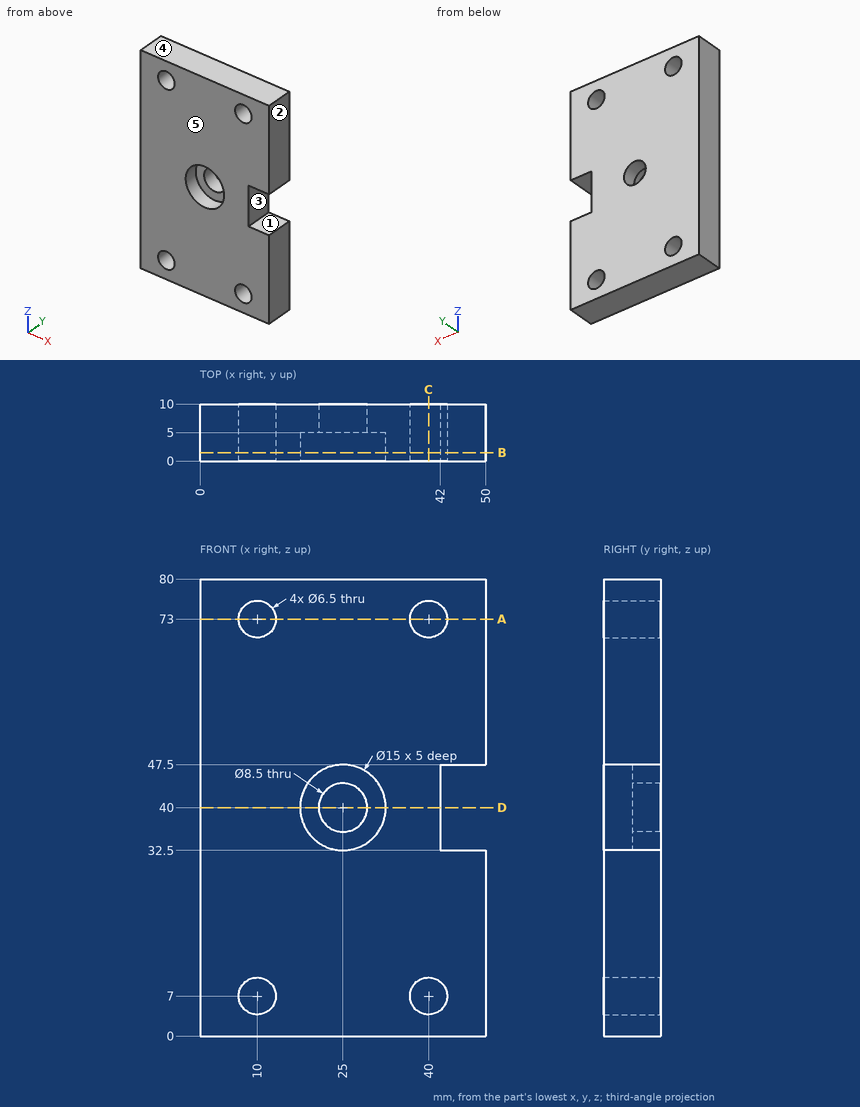
Geometry: see drawing. Coordinates: mm, zero at the bounding-box minimum. A direction names the side the tool comes from. Give positions to 0.01 mm unless a question says otherwise; leave off trailing zeros. Order: outer loops, then holes, each group sorted by start corner. A loop starts at its lowest first (then second) coordinate and runs counter-clockwise, first axis right, second up. Notation, with made-up numbers: (67, -37.75) - (71, -37.75) arc R20 ccw to (71, 0.25) - close; hole circle Ø9 at (-14, 79.25). An arc over 180 degrees is marked (long way). Use CSV: the item, a comma, the result in double quotes.
1. Section query D-D (z = 40). Output: boundary loops of the cut face in (x, y), plus the area to 4 significant figures.
Answers below:
outline,"(0, 0) - (17.5, 0) - (17.5, 5) - (20.75, 5) - (20.75, 10) - (0, 10) - close; (29.25, 5) - (32.5, 5) - (32.5, 0) - (42, 0) - (42, 10) - (29.25, 10) - close"
area,"302.5 mm2"
2. Section query B-B (y = 1.5). Output: boundary loops of the cut face in (x, z), plus the area to 3 significant figures.
Answers below:
outline,"(0, 0) - (50, 0) - (50, 32.5) - (42, 32.5) - (42, 47.5) - (50, 47.5) - (50, 80) - (0, 80) - close; hole circle Ø6.5 at (10, 7); hole circle Ø6.5 at (10, 73); hole circle Ø15 at (25, 40); hole circle Ø6.5 at (40, 7); hole circle Ø6.5 at (40, 73)"
area,"3,570 mm2"
3. Section query A-A (z = 73). Output: boundary loops of the cut face in (x, y), plus the area to 3 significant figures.
Answers below:
outline,"(0, 0) - (6.75, 0) - (6.75, 10) - (0, 10) - close; (13.25, 0) - (36.75, 0) - (36.75, 10) - (13.25, 10) - close; (43.25, 0) - (50, 0) - (50, 10) - (43.25, 10) - close"
area,"370 mm2"
4. Contact query for a flat-ended pin moving along its axis: pin 1 (13.5 mm diameter, centred on x = 25, z = 40, fed in from -Y). Output: stop coordinate, or through.
Answers below:
pin 1,"y = 5"
5. Mould query, pull axis Z, two halves, no side actions, for the marked faces 3, 4 and 5. Classes: +Z half, -Z half, draft (parallel to the pull), parting line (faces both ways), or undercut.
Answers below:
face 3,"undercut"
face 4,"+Z half"
face 5,"draft"
6. Section query C-C (x = 40). Output: boundary loops of the cut face in (y, z), plus the area to 3 significant figures.
Answers below:
outline,"(0, 0) - (10, 0) - (10, 3.75) - (0, 3.75) - close; (0, 10.25) - (10, 10.25) - (10, 69.75) - (0, 69.75) - close; (0, 76.25) - (10, 76.25) - (10, 80) - (0, 80) - close"
area,"670 mm2"
7. Access query for the marked faces 1 and 2. Directions: +Z, -Z, +X, -X, +Y, -Y. A direction counts if a zero-diameter tool reaches every point of the face in a straight line with its end or side. Return the directions, or none.
Answers below:
face 1,"+X, +Y, -Y"
face 2,"+Z, -Z, +X, +Y, -Y"
8. Material intervals for line 1 along X through (y, z) = (5, 7); line 2 along Z through (x, y) = (10, 6.25); line 3 along X through (y, z) = (5, 9), sorted ascending. Write a range as from..to.
Answers below:
line 1,"0..6.75, 13.25..36.75, 43.25..50"
line 2,"0..3.75, 10.25..69.75, 76.25..80"
line 3,"0..7.44, 12.56..37.44, 42.56..50"
